from build123d import *

# Parameters (mm, degrees)
R_P_TITION_CIRCULAIRE1_COUNT = 3


with BuildPart() as part:
    # Esquisse1 → Révolution1 (revolve)
    with BuildSketch(Plane.XY, mode=Mode.PRIVATE) as r_volution1_sk:
        Polygon((23.5, 0), (23.5, 53), (20, 53), (20, 55), (31, 55), (35, 51), (35, 22), (48, 22), (48, 0), align=None)
    revolve(r_volution1_sk.sketch.rotate(Axis((0, 45.247444815, 0), (0, -1, 0)), 90), axis=Axis((0, 45.247444815, 0), (0, -1, 0)))

    # Esquisse2 → Trou taraudé M61 (revolve, cut)
    with BuildSketch(Plane(origin=(43.498358535, 22, -0.377895148), x_dir=(0, 0, 1), z_dir=(1, 0, 0))):
        Polygon((0, 0), (0, 18.443375673), (2.5, 17), (2.5, 0), align=None)
    trou_taraud_m61 = revolve(axis=Axis((43.498358535, 28.35, -0.377895148), (0, -1, 0)), mode=Mode.SUBTRACT)

    # Esquisse3 → Trou taraudé M41 (revolve, cut)
    with BuildSketch(Plane(origin=(28, 0, 0), x_dir=(0, 0, -1), z_dir=(1, 0, 0))):
        Polygon((0, 0), (0, 12.452627944), (1.65, 11.5), (1.65, 0), align=None)
    trou_taraud_m41 = revolve(axis=Axis((28, -6.35, 0), (0, 1, 0)), mode=Mode.SUBTRACT)

    # Esquisse4 → Trou taraudé M62 (revolve, cut)
    with BuildSketch(Plane(origin=(-43, 0, 0), x_dir=(0, 0, -1), z_dir=(1, 0, 0))):
        Polygon((0, 0), (0, 18.443375673), (2.5, 17), (2.5, 0), align=None)
    trou_taraud_m62 = revolve(axis=Axis((-43, -6.35, 0), (0, 1, 0)), mode=Mode.SUBTRACT)

    # Répétition circulaire1: Trou taraudé M61, Trou taraudé M41, Trou taraudé M62 ×3 about axis
    r_p_tition_circulaire1_axis = Axis((0, 0, 0), (0, 1, 0))
    add([trou_taraud_m61.rotate(r_p_tition_circulaire1_axis, i * 360 / R_P_TITION_CIRCULAIRE1_COUNT) for i in range(1, R_P_TITION_CIRCULAIRE1_COUNT)], mode=Mode.SUBTRACT)
    add([trou_taraud_m41.rotate(r_p_tition_circulaire1_axis, i * 360 / R_P_TITION_CIRCULAIRE1_COUNT) for i in range(1, R_P_TITION_CIRCULAIRE1_COUNT)], mode=Mode.SUBTRACT)
    add([trou_taraud_m62.rotate(r_p_tition_circulaire1_axis, i * 360 / R_P_TITION_CIRCULAIRE1_COUNT) for i in range(1, R_P_TITION_CIRCULAIRE1_COUNT)], mode=Mode.SUBTRACT)


solid = part.part
Geometry: final body of the model. Coordinates: model frame, mm. A direction names the side the tool comes from. Coordinates: 2 decimals unless noted, no trailing zeros. Order: outer loops, then holes, each group sorted by start corner. A loop starts at its lowest first (then second) coordinate and runs counter-clockwise, first axis right, second up.
(1) Section query B-B (y = 8). State how many separate pieces and enclosed holes the cut face has, plus the area to 3 significant figures.
(2) Section query A-A (x = 0). Return the cut outline in (y, z), plus the area to 4 significant figures.
(3) Draft query along Z for faces 4 (the face through (-21.65, 3.81, -37.58)), 5 (the face through (-23.3, 26.87, -3.06)), 6 (the face through (-14.418, 10.846, 45.783)), 7 (the face through (21, 0, -11)). Return one class per face: pulls with the +Z half, pulls with the -Z half, needs draft (parallel to the pull), parting line crosses it, or undercut.
(4) Material intervals for probe 1 along X at (y, z) = (4, 0); probe 2 along Y at (x, z) = (12, 37); probe 3 along X at (y, z) = (51, 21), sorted ascending.
(5) Access query for faces 1 (the face through (-18.98, 13.62, 37.32)), 2 (the face through (-0.88, 54.01, -19.98)), 3 (the face through (26.364, 5.67, 0.215)). Directions: +Z, -Z, +X, -X, +Y, -Y. A direction counts if a zero-diameter tool reaches every point of the face in a straight line with its end or side. Return the directions, or none.
(6) First-contact query: pin 1 (10 mm diameter, centred on x = 6, y = 30, fed in from -Z); pin 2 (3 mm diameter, centred on x = -5, y = 44, fed in from -Z); pin 3 (6.5 mm diameter, centred on x = 21.5, z = 37.24, fed in from +Y). Flat tips, straight axial feed; report the tip coordinate or a pass-through.
(7) Section query C-C (y = 37). Return the cut outline in (x, z), plus the area to 3 significant figures.
Solution:
1. separate pieces: 1
1. enclosed holes: 10
1. area: 5,360 mm2
2. outline: (0, -48) - (22, -48) - (22, -35) - (51, -35) - (55, -31) - (55, -20) - (53, -20) - (53, -23.5) - (0, -23.5) - close; (0, 23.5) - (53, 23.5) - (53, 20) - (55, 20) - (55, 31) - (51, 35) - (22, 35) - (22, 48) - (0, 48) - close
2. area: 1,835 mm2
3. face 4: undercut
3. face 5: undercut
3. face 6: parting line crosses it
3. face 7: needs draft
4. probe 1: x = -48 to -45.5, -40.5 to -23.5, 23.5 to 26.35, 29.65 to 42.83, 44.17 to 48
4. probe 2: y = 0 to 22
4. probe 3: x = -28 to -10.55, 10.55 to 28
5. face 1: +Y
5. face 2: +Y, -Y
5. face 3: -Y
6. pin 1: stops at z = -34.99
6. pin 2: stops at z = -34.82
6. pin 3: stops at y = 22
7. outline: circle Ø70 at (0, 0); hole circle Ø47 at (0, 0)
7. area: 2,110 mm2
